Geometry: final body of the model. Coordinates: model frame, mm. A direction names the side the tool comes from. Coordinates: 2 decimals unless noted, no trailing zeros. Write each loop counter-clockwise with the first axis right and the second up, starting at its lowest first coordinate (ties: lowest second). Pieces come first, ordered by that corner, then holes.
from build123d import *

# Parameters (mm, degrees)
SKETCH1_R           = 2.25
BOSS_EXTRUDE1_DEPTH = 45
CHAMFER1_SIZE       = 3.535533906
SKETCH2_W           = 35
SKETCH2_H           = 10.606601718
CUT_EXTRUDE1_DEPTH  = 12.5
CIRPATTERN1_COUNT   = 4


with BuildPart() as part:
    # Sketch1 → Boss-Extrude1 (new body)
    # profile 1 of 12: a face of its own
    with BuildSketch(Plane.XY):
        with BuildLine():
            Line((0, 60), (0, 52.5))
            Line((0, 52.5), (10.010851315, 42.489148685))
            ThreePointArc((10.010851315, 42.489148685), (13.333493167, 46.666506833), (17.510851315, 49.989148685))
            Line((17.510851315, 49.989148685), (7.5, 60))
            Line((7.5, 60), (0, 60))
        make_face()
        with Locations(Location((6.43, 53.57, 0), (0, 0, 180))):
            Circle(SKETCH1_R, mode=Mode.SUBTRACT)
    # profile 2 of 12: a face of its own
    with BuildSketch(Plane.XY):
        with BuildLine():
            ThreePointArc((17.510851315, 49.989148685), (13.333493167, 46.666506833), (10.010851315, 42.489148685))
            Line((10.010851315, 42.489148685), (12.98114549, 39.51885451))
            ThreePointArc((12.98114549, 39.51885451), (16.211417767, 43.788582233), (20.48114549, 47.01885451))
            Line((20.48114549, 47.01885451), (17.510851315, 49.989148685))
        make_face()
    # profile 3 of 12: a face of its own
    with BuildSketch(Plane.XY):
        with BuildLine():
            ThreePointArc((42.489148685, 49.989148685), (30, 53.57), (17.510851315, 49.989148685))
            Line((17.510851315, 49.989148685), (20.48114549, 47.01885451))
            ThreePointArc((20.48114549, 47.01885451), (30, 49.5), (39.51885451, 47.01885451))
            Line((39.51885451, 47.01885451), (42.489148685, 49.989148685))
        make_face()
    # profile 4 of 12: a face of its own
    with BuildSketch(Plane.XY):
        with BuildLine():
            ThreePointArc((49.989148685, 42.489148685), (46.666506833, 46.666506833), (42.489148685, 49.989148685))
            Line((42.489148685, 49.989148685), (39.51885451, 47.01885451))
            ThreePointArc((39.51885451, 47.01885451), (43.788582233, 43.788582233), (47.01885451, 39.51885451))
            Line((47.01885451, 39.51885451), (49.989148685, 42.489148685))
        make_face()
    # profile 5 of 12: a face of its own
    with BuildSketch(Plane.XY):
        with BuildLine():
            Line((49.989148685, 42.489148685), (60, 52.5))
            Line((60, 52.5), (60, 60))
            Line((60, 60), (52.5, 60))
            Line((52.5, 60), (42.489148685, 49.989148685))
            ThreePointArc((42.489148685, 49.989148685), (46.666506833, 46.666506833), (49.989148685, 42.489148685))
        make_face()
        with Locations(Location((53.57, 53.57, 0), (0, 0, 180))):
            Circle(SKETCH1_R, mode=Mode.SUBTRACT)
    # profile 6 of 12: a face of its own
    with BuildSketch(Plane.XY):
        with BuildLine():
            Line((47.01885451, 20.48114549), (49.989148685, 17.510851315))
            ThreePointArc((49.989148685, 17.510851315), (52.657108537, 23.503821681), (53.57, 30))
            ThreePointArc((53.57, 30), (52.657108537, 36.496178319), (49.989148685, 42.489148685))
            Line((49.989148685, 42.489148685), (47.01885451, 39.51885451))
            ThreePointArc((47.01885451, 39.51885451), (48.869521231, 34.918451843), (49.5, 30))
            ThreePointArc((49.5, 30), (48.869521231, 25.081548157), (47.01885451, 20.48114549))
        make_face()
    # profile 7 of 12: a face of its own
    with BuildSketch(Plane.XY):
        with BuildLine():
            Line((42.489148685, 10.010851315), (52.5, 0))
            Line((52.5, 0), (60, 0))
            Line((60, 0), (60, 7.5))
            Line((60, 7.5), (49.989148685, 17.510851315))
            ThreePointArc((49.989148685, 17.510851315), (46.666506833, 13.333493167), (42.489148685, 10.010851315))
        make_face()
        with Locations(Location((53.57, 6.43, 0), (0, 0, 180))):
            Circle(SKETCH1_R, mode=Mode.SUBTRACT)
    # profile 8 of 12: a face of its own
    with BuildSketch(Plane.XY):
        with BuildLine():
            Line((20.48114549, 12.98114549), (17.510851315, 10.010851315))
            ThreePointArc((17.510851315, 10.010851315), (30, 6.43), (42.489148685, 10.010851315))
            Line((42.489148685, 10.010851315), (39.51885451, 12.98114549))
            ThreePointArc((39.51885451, 12.98114549), (30, 10.5), (20.48114549, 12.98114549))
        make_face()
    # profile 9 of 12: a face of its own
    with BuildSketch(Plane.XY):
        with BuildLine():
            ThreePointArc((10.010851315, 17.510851315), (13.333493167, 13.333493167), (17.510851315, 10.010851315))
            Line((17.510851315, 10.010851315), (20.48114549, 12.98114549))
            ThreePointArc((20.48114549, 12.98114549), (16.211417767, 16.211417767), (12.98114549, 20.48114549))
            Line((12.98114549, 20.48114549), (10.010851315, 17.510851315))
        make_face()
    # profile 10 of 12: a face of its own
    with BuildSketch(Plane.XY):
        with BuildLine():
            Line((0, 7.5), (0, 0))
            Line((0, 0), (7.5, 0))
            Line((7.5, 0), (17.510851315, 10.010851315))
            ThreePointArc((17.510851315, 10.010851315), (13.333493167, 13.333493167), (10.010851315, 17.510851315))
            Line((10.010851315, 17.510851315), (0, 7.5))
        make_face()
        with Locations(Location((6.43, 6.43, 0), (0, 0, 180))):
            Circle(SKETCH1_R, mode=Mode.SUBTRACT)
    # profile 11 of 12: a face of its own
    with BuildSketch(Plane.XY):
        with BuildLine():
            Line((39.51885451, 12.98114549), (42.489148685, 10.010851315))
            ThreePointArc((42.489148685, 10.010851315), (46.666506833, 13.333493167), (49.989148685, 17.510851315))
            Line((49.989148685, 17.510851315), (47.01885451, 20.48114549))
            ThreePointArc((47.01885451, 20.48114549), (43.788582233, 16.211417767), (39.51885451, 12.98114549))
        make_face()
    # profile 12 of 12: a face of its own
    with BuildSketch(Plane.XY):
        with BuildLine():
            ThreePointArc((10.010851315, 42.489148685), (6.43, 30), (10.010851315, 17.510851315))
            Line((10.010851315, 17.510851315), (12.98114549, 20.48114549))
            ThreePointArc((12.98114549, 20.48114549), (10.5, 30), (12.98114549, 39.51885451))
            Line((12.98114549, 39.51885451), (10.010851315, 42.489148685))
        make_face()
    extrude(amount=BOSS_EXTRUDE1_DEPTH)

    # Chamfer1
    chamfer1_edges = [part.edges().sort_by_distance(p)[0] for p in [
        (0, 60, 22.5),
        (60, 60, 22.5),
        (60, 0, 22.5),
        (0, 0, 22.5),
    ]]
    chamfer(chamfer1_edges, length=CHAMFER1_SIZE)

    # Sketch2 → Cut-Extrude1 (cut)
    with BuildSketch(Plane(origin=(58.232233047, 58.232233047, 0), x_dir=(0, 0, -1), z_dir=(0.7071067811865489, 0.7071067811865461, 0))):
        with Locations((-22.5, 0)):
            Rectangle(SKETCH2_W, SKETCH2_H)
    cut_extrude1 = extrude(amount=-CUT_EXTRUDE1_DEPTH, mode=Mode.SUBTRACT)

    # CirPattern1: Cut-Extrude1 ×4 about axis
    cirpattern1_axis = Axis((30, 30, 0), (0, 0, 1))
    for i in range(1, CIRPATTERN1_COUNT):
        add(cut_extrude1.rotate(cirpattern1_axis, i * 360 / CIRPATTERN1_COUNT), mode=Mode.SUBTRACT)


solid = part.part
Item 1: Set-up query: faces 1 (the flat face through (56, 52, 5)), 2 (the flat face through (14.8, 52.7, 22.2)), 3 (the flat face through (45.2, 7.3, 22.2)). Return all of +Z, -Z, +X, -X, +Y, -Y with unobstructed straight access to the full face (end or side cutting, diameter ignored); none if empty.
Derived:
face 1: +X, +Y
face 2: +Z, -Z, +Y
face 3: +Z, -Z, -Y
Item 2: Section A-A, the plane y = 25.5. Output: boundary loops of the cut face in (x, z), plus the area to 3 significant figures.
Derived:
outline: (6.86, 0) - (11.03, 0) - (11.03, 45) - (6.86, 45) - close; (48.97, 0) - (53.14, 0) - (53.14, 45) - (48.97, 45) - close
area: 375 mm2
Item 3: Pin query (flat end, axial travel): pin 1 (6 mm diameter, centred on y = 48.5, z = 23, fed in from -X); pin 2 (1 mm diameter, centred on y = 24.5, z = 36, fed in from +X); pin 3 (5 mm diameter, centred on x = 6.43, y = 53.57, fed in from +Z); pin 4 (6 mm diameter, centred on y = 37, z = 39.5, fed in from -X). Return the tip coordinate at first contact, or that it passes through.
Derived:
pin 1: stops at x = 6.86
pin 2: stops at x = 53.03
pin 3: stops at z = 45
pin 4: stops at x = 6.77
Item 4: Section C-C, the plane x = 15.5. Output: boundary loops of the cut face in (y, z), plus the area to 3 significant figures.
Derived:
outline: (8, 0) - (16.96, 0) - (16.96, 45) - (8, 45) - close; (43.04, 0) - (52, 0) - (52, 45) - (43.04, 45) - close
area: 807 mm2
Item 5: Material intervals for probe 1 along X at (y, z) = (6, 42); probe 2 along Y at (x, z) = (5.5, 41.5), sorted ascending.
Derived:
probe 1: x = 0 to 4.22, 8.64 to 13.5, 46.5 to 51.36, 55.78 to 60
probe 2: y = 0 to 4.38, 8.48 to 13, 47 to 51.52, 55.62 to 60
Item 6: Section B-B, the plane z = 17.5. Output: boundary loops of the cut face in (x, y), plus the area to 3 significant figures.
Derived:
outline: (6.86, 14.36) - (14.36, 6.86) - (17.51, 10.01) arc R23.57 ccw to (42.49, 10.01) - (45.64, 6.86) - (53.14, 14.36) - (49.99, 17.51) arc R23.57 ccw to (49.99, 42.49) - (53.14, 45.64) - (45.64, 53.14) - (42.49, 49.99) arc R23.57 ccw to (17.51, 49.99) - (14.36, 53.14) - (6.86, 45.64) - (10.01, 42.49) arc R23.57 ccw to (10.01, 17.51) - close; hole circle Ø39 at (30, 30)
area: 723 mm2
Item 7: Pull-direction query (Z, two-part tool) for faces 4 (the flat face through (7.3, 14.8, 22.2)), 5 (the flat face through (56, 52, 40)); classes: released by +Z, released by -Z, zero draft, split by the parting line, or undercut.
Derived:
face 4: zero draft
face 5: undercut
Item 8: Section D-D, the plane y = 48.5. Output: boundary loops of the cut face in (x, z).
Derived:
outline: (4, 0) - (23.84, 0) - (23.84, 45) - (4, 45) - (4, 40) - (9.71, 40) - (9.71, 5) - (4, 5) - close; (36.16, 0) - (56, 0) - (56, 5) - (50.29, 5) - (50.29, 40) - (56, 40) - (56, 45) - (36.16, 45) - close
